Geometry check sheet. Reference: drawing and pictorial views, mm from the part's lowest x, y, z. Give positions to 0.01 mm unless a question says otherwise; leave off trailing zeros. Order: outer loops, then holes, each group sorted by start corner. A loop starts at its lowest first (then second) coordinate and runs counter-clockwise, first axis right, second up.
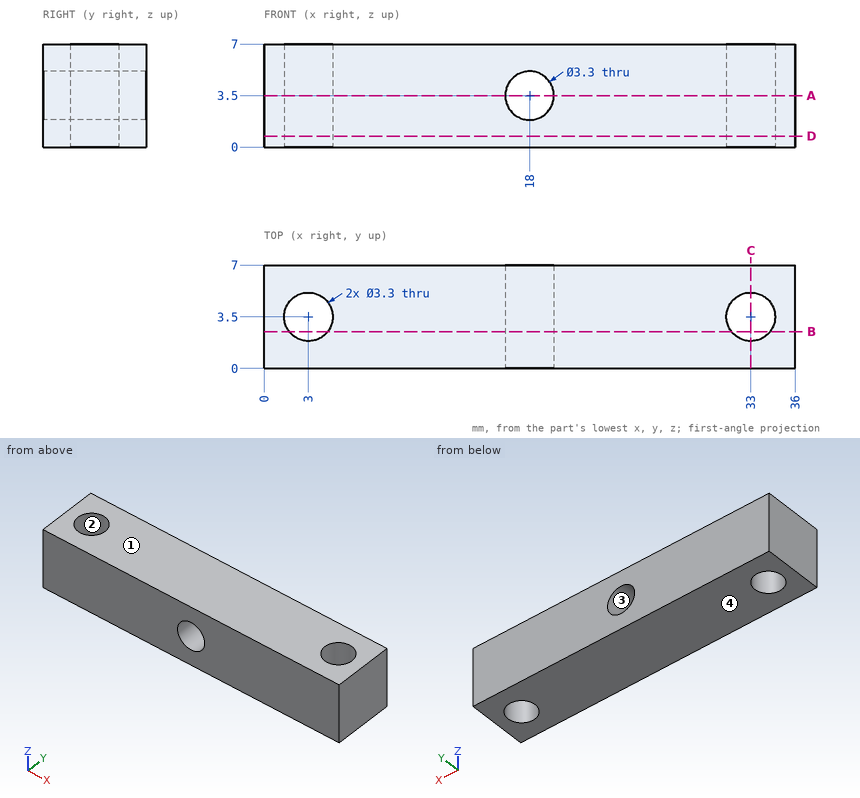
(1) Thickness scan on L1, parallel to Y at x = 33, z = 2; L2, parallel to X at y = 3.25, z = 0.75. Record the ranges inside material, lowest first.
(2) Sectioned sample at D-D (z = 0.75). Enter the section's corners in (x, y).
(3) Sectioned sample at B-B (y = 2.5). Enter the section's corners in (x, z).
(4) Release check for a two-part mould opening along Z. For the marked faces 1, 2, 3 and 4 record: released by +Z, released by -Z, zero draft, split by the parting line, or undercut.
(5) Sectioned sample at A-A (z = 3.5). Enter the section's corners in (x, y), plus the area to 3 significant figures.
(6) Sectioned sample at C-C (x = 33). Enter the section's corners in (y, z), plus the area to 3 significant figures.
Values follow:
1. L1: y = 0 to 1.85, 5.15 to 7
1. L2: x = 0 to 1.37, 4.63 to 31.37, 34.63 to 36
2. outline: (0, 0) - (36, 0) - (36, 7) - (0, 7) - close; hole circle Ø3.3 at (3, 3.5); hole circle Ø3.3 at (33, 3.5)
3. outline: (0, 0) - (1.69, 0) - (1.69, 7) - (0, 7) - close; (4.31, 0) - (31.69, 0) - (31.69, 7) - (4.31, 7) - close; (34.31, 0) - (36, 0) - (36, 7) - (34.31, 7) - close; hole circle Ø3.3 at (18, 3.5)
4. face 1: released by +Z
4. face 2: zero draft
4. face 3: undercut
4. face 4: released by -Z
5. outline: (0, 0) - (16.35, 0) - (16.35, 7) - (0, 7) - close; (19.65, 0) - (36, 0) - (36, 7) - (19.65, 7) - close; hole circle Ø3.3 at (3, 3.5); hole circle Ø3.3 at (33, 3.5)
5. area: 212 mm2
6. outline: (0, 0) - (1.85, 0) - (1.85, 7) - (0, 7) - close; (5.15, 0) - (7, 0) - (7, 7) - (5.15, 7) - close
6. area: 25.9 mm2
